Answer from the drawing. Dimensions are ordinates in mm from the lowest x, y and z of the part. A direction names the side the tool comes from. Coordinates: 2 decimals unless noted, no trailing zeros. Write each loop counter-clockwise with the first axis right and the second up, starting at its lowest first coordinate (ties: lowest second). Pieces come first, ordered by that corner, then holes.
(1) Find the intervals of material crossed by probe 1 along Z at (x, y) = (21.5, 42); probe 2 along Y at (x, z) = (14, 11) (1 decimal); probe 3 along Y at (x, z) = (40, 9.25), in increasing order.
(2) Section C-C on z = 10.75 is taken. Write down the section's boundary in (x, y) (1 decimal), then the cut area to 4 significant figures.
(3) The mould has two halves that part along X. Classify the marked faces 4, 5 and 6: +X half, -X half, draft (parallel to the pull), parting line (faces both ways), or undercut.
(4) Given pin 1 (1.5 mm diameter, centred on x = 36.5, z = 10.5, fed in from -Y) (1 decimal); pin 2 (1.5 mm diameter, centred on y = 54.5, z = 4, fed in from +X); pin 3 (4 mm diameter, centred on x = 37, y = 34, fed in from -Z), each flat-ended and moving along its own axis, determine where each tip first touches the part or whether it passes through.
(5) Which of the six approach directions +Z, -Z, +X, -X, +Y, -Y give full straight-line access (tool end or side, diameter ignored) to the marked faces 1, 2 and 3?
(6) Section A-A on z = 4.5 is taken. Write down the section's boundary in (x, y) (1 decimal).
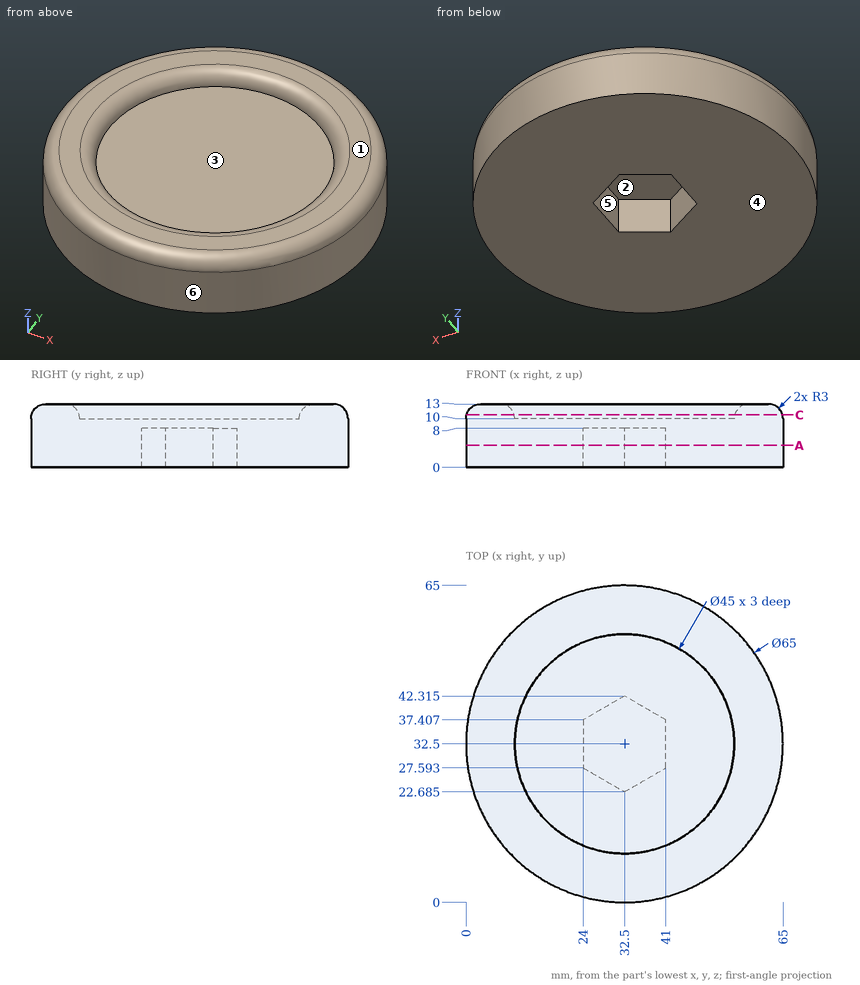
Response:
1. probe 1: z = 0 to 10
1. probe 2: y = 6 to 19.4, 45.6 to 59
1. probe 3: y = 0.88 to 64.12
2. outline: circle Ø64.8 at (32.5, 32.5); hole circle Ø45.2 at (32.5, 32.5)
2. area: 1,695 mm2
3. face 4: draft
3. face 5: undercut
3. face 6: parting line
4. pin 1: stops at y = 0.2
4. pin 2: stops at x = 57.09
4. pin 3: stops at z = 8
5. face 1: +Z, +X, -X, +Y, -Y
5. face 2: -Z
5. face 3: +Z
6. outline: circle Ø65 at (32.5, 32.5); hole (24, 27.6) - (32.5, 22.7) - (41, 27.6) - (41, 37.4) - (32.5, 42.3) - (24, 37.4) - close
